```python
from build123d import *

# Parameters (mm, degrees)
F0_R     = 15.875
F1_DEPTH = 25.4
F2_D     = 10.3
F3_SIZE  = 0.79375
F4_SIZE  = 0.79375
F5_R     = 15.875
F5_R_2   = 7.9375
F6_DEPTH = 19.05
F7_SIZE  = 0.79375


with BuildPart() as f1:
    # F0 (on Top) → F1 (new body)
    with BuildSketch(Plane.XY):
        Circle(F0_R)
    extrude(amount=F1_DEPTH)

    # F2 (through all)
    with Locations(Plane(origin=(0, 0, 0), x_dir=(1, 0, 0), z_dir=(0, 0, -1))):
        with Locations((0, 0)):
            Hole(F2_D / 2)

    # F3
    f3_edges = [f1.edges().sort_by_distance(p)[0] for p in [
        (-15.875, 0, 0),
    ]]
    chamfer(f3_edges, length=F3_SIZE)

    # F4
    f4_edges = [f1.edges().sort_by_distance(p)[0] for p in [
        (-15.875, 0, 25.4),
        (-5.15, 0, 25.4),
        (-5.15, 0, 0),
    ]]
    chamfer(f4_edges, length=F4_SIZE)

    # F5 (on face) → F6 (cut)
    with BuildSketch(Plane.XY.offset(25.4)):
        Circle(F5_R)
        Circle(F5_R_2, mode=Mode.SUBTRACT)
    extrude(amount=-F6_DEPTH, mode=Mode.SUBTRACT)

    # F7
    f7_edges = [f1.edges().sort_by_distance(p)[0] for p in [
        (-15.875, 0, 6.35),
        (-7.9375, 0, 6.35),
        (-7.9375, 0, 25.4),
    ]]
    chamfer(f7_edges, length=F7_SIZE)


solid = f1.part
```
CAD build for the part. Positions are in the model's coordinates, mm. A direction names the side the tool comes from. Coordinates: 2 decimals unless noted, no trailing zeros. Write each loop counter-clockwise with the first axis right and the second up, starting at its lowest first coordinate (ties: lowest second). Pieces come first, ordered by that corner, then holes. Notation, with made-up numbers: (-13.75, 15) -> (25.25, 15) arc R11 cw to (25.25, 31) -> close; hole circle Ø11 at (-32.75, -25). An arc over 180 degrees is marked (long way). Return JSON: item names as keys, results as strings. Group by question number.
Q1. Which spindle directions (+Z, -Z, +X, -X, +Y, -Y) get a long thin tool onto all of the face, cutting with end or side? Do faces 4 (the face through (-1.72, -7.75, 16)), 5 (the face through (-0.2, -6.5, 0)). Say none if no direction does.
Q2. Cut at D-D, the plane z = 2.5. Give the cut face in (x, y) (3 decimals), then the cut area to 3 significant figures.
Q3. Pull direction Y, two halves, no side cores. Call faces 1 (the face through (-2, 6, 25.4)), 2 (the face through (-3.441, -15.497, 3.142)), 3 (the face through (-4.91, -1.55, 12.87)): released by +Y, released by -Y, zero draft, split by the parting line, or undercut.
Q4. Flat gauge pins, fed straight in: pin 1 (8 mm diameter, centred on x = 6, z = 3, fed in from +Y); pin 2 (4 mm diameter, centred on y = 7.5, z = 6.5, fed in from -X); pin 3 (8 mm diameter, centred on x = 6, z = 13.5, fed in from +Y). Where does each tip first touch, or does it go through?
Q5. Drill centre lines: line 1 (Y direction, x = 0, z = 9.25); line 2 (Z direction, x = -8, y = -3.5); line 3 (Y direction, x = -4, z = 23.25). Where is each one in solid material? Low to high.
Returned:
{
 "1": {"face 4": "+Z", "face 5": "-Z, +X, -X, +Y, -Y"},
 "2": {"outline": "circle Ø31.75 at (0, 0); hole circle Ø10.3 at (0, 0)", "area": "708 mm2"},
 "3": {"face 1": "zero draft", "face 2": "split by the parting line", "face 3": "undercut"},
 "4": {"pin 1": "stops at y = 15.75", "pin 2": "stops at x = -14.8", "pin 3": "stops at y = 7.68"},
 "5": {"line 1": "y = -7.94 to -5.15, 5.15 to 7.94", "line 2": "z = 0 to 6.35", "line 3": "y = -6.86 to -3.24, 3.24 to 6.86"}
}
